Read the model definition and answer for the solid it produces. Units are mm, in the model's axes. A direction names the side the tool comes from. Coordinates: 2 decimals unless noted, no trailing zeros. Loops run counter-clockwise (first coordinate to the right, second up) from the corner with the lowest first, then second, coordinate; pieces in that order, holes last.
Q1. Section A-A (z = 65.5) is taken. Give the vertices of the cut face in (x, y).
Q2. Section C-C (x = -41.5) is taken. Give the vertices of the cut face in (y, z).
Q3. Section B-B (y = -105.5) is taken. Give the vertices of the cut face in (x, z), then the cut area to 3 significant figures.
Q4. Flat-ended cylindrical pins translate along their axes: P1, Ø20, axis at x = 37.5, z = 75, coming from the +Y side; P2, Ø20, axis at x = 32, z = 19.5, coming from the -Y side; P3, Ø5, axis at y = -92.5, z = -73, coming from the +X side. Find the tip coordinate at first contact, or state that the pin passes through.
Q5. Which of the six approach directions +Z, -Z, +X, -X, +Y, -Y give full straight-line access (tool end or side, diameter ignored) to faces 1 (the face through (-10, 101, 2)), 2 (the face through (10, 101, 2)), 3 (the face through (-10, -99, 2)), 4 (the face through (30, -50, 2))?
Q6. Straight lines are drawn through the part: line 1 (X direction, y = 96, z = -131); line 2 (Y direction, x = 22, z = -129.5). For each, find the intervals that lie inside material, in ascending order.
from build123d import *

# Parameters (mm, degrees)
SKETCH3_W           = 300
SKETCH3_H           = 100
BOSS_EXTRUDE3_DEPTH = 50
SKETCH3_4_W         = 300
SKETCH3_4_H         = 100
BOSS_EXTRUDE4_DEPTH = 10


with BuildPart() as part:
    # Sketch3 → Boss-Extrude3 (new, symmetric)
    with BuildSketch(Plane(origin=(0, 0, 0), x_dir=(0, 0, -1), z_dir=(1, 0, 0))):
        Rectangle(SKETCH3_W, SKETCH3_H)
    extrude(amount=BOSS_EXTRUDE3_DEPTH, both=True)

    # Sketch3<4> → Boss-Extrude4 (add, symmetric)
    with BuildSketch(Plane(origin=(0, 0, 0), x_dir=(0, 0, -1), z_dir=(1, 0, 0))):
        with Locations((0, 100)):
            Rectangle(SKETCH3_4_W, SKETCH3_4_H)
        with Locations((0, -100)):
            Rectangle(SKETCH3_4_W, SKETCH3_4_H)
    extrude(amount=BOSS_EXTRUDE4_DEPTH, both=True)


solid = part.part
Numbers:
1. outline: (-50, -50) - (-10, -50) - (-10, -150) - (10, -150) - (10, -50) - (50, -50) - (50, 50) - (10, 50) - (10, 150) - (-10, 150) - (-10, 50) - (-50, 50) - close
2. outline: (-50, -150) - (50, -150) - (50, 150) - (-50, 150) - close
3. outline: (-10, -150) - (10, -150) - (10, 150) - (-10, 150) - close
3. area: 6,000 mm2
4. P1: stops at y = 50
4. P2: stops at y = -50
4. P3: stops at x = 10
5. face 1: +Z, -Z, -X, +Y
5. face 2: +Z, -Z, +X, +Y
5. face 3: +Z, -Z, -X, -Y
5. face 4: +Z, -Z, +X, -Y
6. line 1: x = -10 to 10
6. line 2: y = -50 to 50
